Can you work these out from the model? Positions are in its coordinate system, mm. Face numbers are marked on the shaded views. Give positions to 0.01 mm unless a question says otherwise; leave off trailing zeros. Loops run counter-clockwise (first coordinate to the right, second up) from the corner with the lowest first, then second, coordinate; pieces in that order, holes last. Notation, with made-up numbers: (17, 32) - (57, 32) arc R29 ccw to (57, 62) - close; hole circle Ø10 at (6.5, -20). An arc over 180 degrees is marked (long way). Answer as a JSON object with one key per item and string values.
Autodesk Inventor part; units mm, degrees
ref_plane "YZ Plane" through (0, 0, 0) normal (1, 0, 0) x (0, 1, 0)
ref_plane "XZ Plane" through (0, 0, 0) normal (0, 1, 0) x (-1, 0, 0)
ref_plane "XY Plane" through (0, 0, 0) normal (0, 0, 1) x (1, 0, 0)
sketch "Sketch1" plane through (0, 0, 0) normal (0, 0, 1) x (1, 0, 0)
  arc A0 (-163.6506, -118.3654) -> (-93.4502, -160) centre (-93.4502, -80) ccw
  line L0 (-92.0944, 160) -> (0, 160)
  line L1 (0, 160) -> (-92.0944, 160)
  arc A1 (0, 160) -> (-51.3175, -151.5471) centre (426.5438, -70.2596) ccw
  arc A2 (-51.3175, -151.5471) -> (-25.1411, -158.0124) centre (0, 0) ccw
  arc A3 (0, 160) -> (-25.1411, -158.0124) centre (0, 0) ccw
  line L2 (-93.4502, -160) -> (-25.2982, -160)
  arc A4 (-25.2982, -160) -> (-25.1411, -158.0124) centre (-25.2982, -159) ccw
  line L3 (-25.2982, -160) -> (-93.4502, -160)
  arc A5 (-163.6506, -118.3654) -> (-93.4502, -160) centre (-93.4502, -80) ccw
  arc A6 (-163.6414, 118.3822) -> (-163.6506, -118.3654) centre (52.9327, 0) ccw
  arc A7 (-92.0944, 160) -> (-163.6414, 118.3822) centre (-93.444, 80.0114) ccw
  point P0 (-51.3175, -151.5471)
  dimension "d53" = 160
  dimension "d55" = 68.152
  dimension "d56" = 80
  dimension "d60" = 92.0944
  dimension "d65" = 1
  dimension "d66" = 484.7258
  dimension "d71" = 246.8171
  dimension "d72" = 80
extrude "Extrusion1" add sketch "Sketch1" along normal mid plane 442.6 contours A6 A7 L0 A3 A2 A4 L2 A0
sketch "Sketch2" plane through (0, 0, 221.3) normal (0, 0, 1) x (1, 0, 0)
  arc A0 (-51.3175, -151.5471) -> (-25.1411, -158.0124) centre (0, 0) ccw
  line L0 (-25.2982, -160) -> (-93.4502, -160)
  arc A1 (-25.2982, -160) -> (-25.1411, -158.0124) centre (-25.2982, -159) ccw
  line L1 (-93.4502, -160) -> (-25.2982, -160)
  arc A2 (-163.6506, -118.3654) -> (-93.4502, -160) centre (-93.4502, -80) ccw
  arc A3 (-163.6506, -118.3654) -> (-93.4502, -160) centre (-93.4502, -80) ccw
  line L2 (-92.0944, 160) -> (0, 160)
  line L3 (0, 160) -> (-92.0944, 160)
  arc A4 (0, 160) -> (-51.3175, -151.5471) centre (426.5438, -70.2596) ccw
  arc A5 (0, 160) -> (-25.1411, -158.0124) centre (0, 0) ccw
  arc A6 (-163.6414, 118.3822) -> (-163.6506, -118.3654) centre (52.9327, 0) ccw
  arc A7 (-92.0944, 160) -> (-163.6414, 118.3822) centre (-93.444, 80.0114) ccw
  dimension "d73" = 160
  dimension "d74" = 68.152
  dimension "d75" = 80
  dimension "d76" = 92.0944
  dimension "d77" = 1
  dimension "d78" = 484.7258
  dimension "d79" = 246.8171
  dimension "d80" = 80
extrude "Extrusion2" add sketch "Sketch2" along normal blind 10
sketch "Sketch10" plane through (0, 0, 231.3) normal (0, 0, 1) x (1, 0, 0)
  circle A0 centre (-125.0944, -30) radius 9
  line L0 (-93.4502, -160) -> (-25.2982, -160)
  arc A1 (-25.2982, -160) -> (-25.1411, -158.0124) centre (-25.2982, -159) ccw
  point P0 (0, 0)
  dimension "d81" = 18
  dimension "d82" = 130
  dimension "d83" = 99.7962
extrude "Extrusion9" add sketch "Sketch10" along normal blind 9.7
mirror "Mirror4" about plane through (0, 0, 0) normal (0, 0, 1) of "Extrusion2", "Extrusion9"
properties part number "Shovel"
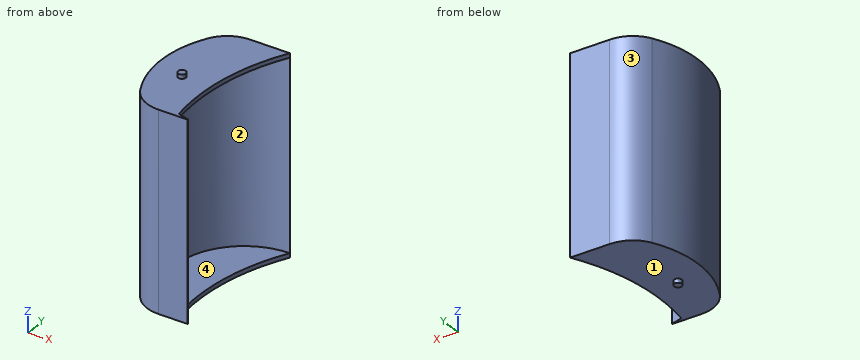
1) I need wall thicknesses on L1, parallel to Z at x = -80, y = -93; L2, parallel to Z at x = -118, y = -26.5; L3, parallel to Z at x = -145, y = -103.5. Which ranges of each line are inside material? Lowest first, please.
Check sheet entries:
{"L1": "-231.3 to -221.3, 221.3 to 231.3", "L2": "-241 to -221.3, 221.3 to 241", "L3": "-231.3 to 231.3"}
2) Imagine slicing it at C-C on z = -91. Write out the boundary of the cut face in (x, y), and give its area (3 significant figures).
Check sheet entries:
{"outline": "(-163.65, -118.37) arc R80 ccw to (-93.45, -160) - (-25.3, -160) arc R1 ccw to (-25.14, -158.01) arc R159.99 cw to (-51.32, -151.55) arc R160 cw to (0, 160) - (-92.09, 160) arc R80 ccw to (-163.64, 118.38) arc R246.82 ccw to start", "area": "15,300 mm2"}
3) Imagine slicing it at B-B on x = -145.5. Write out the boundary of the cut face in (y, z).
Check sheet entries:
{"outline": "(-140.75, -231.3) - (140.76, -231.3) - (140.76, 231.3) - (-140.75, 231.3) - close; hole (-66.56, -221.3) - (66.56, -221.3) - (66.56, 221.3) - (-66.56, 221.3) - close"}
4) Imagine slicing it at A-A on y = 112. Write out the boundary of the cut face in (x, z).
Check sheet entries:
{"outline": "(-167.01, -231.3) - (-22.61, -231.3) - (-22.61, -221.3) - (-114.26, -221.3) - (-114.26, 221.3) - (-22.61, 221.3) - (-22.61, 231.3) - (-167.01, 231.3) - close"}
5) I'm going to push flat-ended pins straight in: P1, Ø5, axis at y = -68, z = -151, coming from the +X side; P2, Ø8, axis at y = -17, z = -109.5, coming from the +X side; P3, Ø1.5, axis at x = -63.5, y = 107.5, coming from the -Z side. Where does each tip first touch, or does it pass through?
Check sheet entries:
{"P1": "x = -143.63", "P2": "x = -158.62", "P3": "z = -231.3"}
6) If we mould it in two halves opening along Y, with no side actions, what happens to the marked faces 1, 2, 3 and 4? For each: released by +Y, released by -Y, zero draft, split by the parting line, or undercut.
Check sheet entries:
{"face 1": "zero draft", "face 2": "undercut", "face 3": "released by +Y", "face 4": "undercut"}
7) Imagine slicing it at D-D on y = -30. Write out the boundary of the cut face in (x, z), and give its area (3 significant figures).
Check sheet entries:
{"outline": "(-192.05, -231.3) - (-134.09, -231.3) - (-134.09, -241) - (-116.09, -241) - (-116.09, -231.3) - (-56.51, -231.3) - (-56.51, -221.3) - (-157.16, -221.3) - (-157.16, 221.3) - (-56.51, 221.3) - (-56.51, 231.3) - (-116.09, 231.3) - (-116.09, 241) - (-134.09, 241) - (-134.09, 231.3) - (-192.05, 231.3) - close", "area": "18,500 mm2"}
